Geometry check sheet. Reference: the model listing, model coordinates, mm. A direction names the side the tool comes from. Round coordinates to 2 decimals unless told otherwise and drop trailing zeros. Write each loop counter-clockwise with the first axis right and the second up, starting at its lowest first coordinate (ties: lowest second). Pieces come first, ordered by that corner, then holes. Notation, with made-up numbers: M 48.5,79 L 73.5,79 A20 cw 73.5,94 Z; hole C -8,20 d5. An arc over 180 degrees is marked long. One line per item, written item: value. Start each with the question number.
1. Depth check by flat-ended pin: P1, Ø1.5, axis at y = 24, z = 2.5, coming from the +X side; P2, Ø1.5, axis at y = 36.5, z = 1, coming from the -X side; P3, Ø2, axis at x = 2.5, z = 2, coming from the +Y side. Enter the tip coordinate at first touch or a pass-through.
2. Section check A-A (z = 1.9). Count the separate pieces of the cut face and the enclosed holes in it, and give its area (3 significant figures).
3. Release check for a two-part mould opening along X. For faces 4 (the cylindrical face through (-14.492, 20.606, 1.972)), 5 (the flat face through (0, -7, 2)), 6 (the cylindrical face through (-7.364, 86.072, 1.972)) record: pulls with the +X half, pulls with the -X half, needs draft (parallel to the pull), parting line crosses it, or undercut.
4. Section check C-C (x = -15.5). Record the boundary of the cut face in (y, z).
5. Access from +Z, -Z, +X, -X, +Y, -Y to the whole of each face (thin tool, end or side, straight path). Record for faces 1 (the cylindrical face through (9.16, 8.95, 1.97)), 2 (the cylindrical face through (-13.47, 81.37, 1.97)), 3 (the flat face through (0, 40, 0)).
6. Scan lines: probe 1 along Y at (x, z) = (-13, 1.8); probe 2 along Y at (x, z) = (4, 1.2); probe 3 along X at (y, z) = (26, 2.2). Record each from-to range of solid material in increasing order. Write a range as [from, to].
7. Section check D-D (y = 62). Record the boundary of the cut face in (x, z), and give its area (3 significant figures).
8. Section check B-B (y = 9.5). Record the boundary of the cut face in (x, z), and give its area (3 significant figures).
from build123d import *

# Parameters (mm, degrees)
SKETCH_1_R          = 3
SKETCH_1_R_2        = 7.5
SKETCH_1_R_3        = 6
EXTRUDE_1_DEPTH     = 4
CUT_EXTRUDE_START   = -10
CUT_EXTRUDE_2_DEPTH = 10
CUT_EXTRUDE_6_DEPTH = 10
FILLET_8_R          = 3
FILLET_9_R          = 10


with BuildPart() as part:
    # 草图1 → 凸台-拉伸1 (new body)
    with BuildSketch(Plane.XY):
        with BuildLine():
            Line((-39.588006912, 70.159203728), (-18.211604838, -1.988557391))
            ThreePointArc((-18.211604838, -1.988557391), (-15.688084184, -5.608917085), (-11.5, -7))
            Line((-11.5, -7), (11.5, -7))
            ThreePointArc((11.5, -7), (16.566581898, -4.83008777), (18.492010075, 0.334357752))
            Line((18.492010075, 0.334357752), (14.982878733, 73.716480896))
            ThreePointArc((14.982878733, 73.716480896), (9.406006267, 84.684478854), (-2.5, 87.790199458))
            Line((-2.5, 87.790199458), (-31.666666667, 82.860132972))
            ThreePointArc((-31.666666667, 82.860132972), (-38.485005613, 78.291944798), (-39.588006912, 70.159203728))
        make_face()
        with Locations((11.5, 0)):
            Circle(SKETCH_1_R, mode=Mode.SUBTRACT)
        with Locations((-11.5, 0)):
            Circle(SKETCH_1_R, mode=Mode.SUBTRACT)
        with Locations((0, 73)):
            Circle(SKETCH_1_R_2, mode=Mode.SUBTRACT)
        with Locations((-30, 73)):
            Circle(SKETCH_1_R_3, mode=Mode.SUBTRACT)
    extrude(amount=EXTRUDE_1_DEPTH)

    # 草图3 → 切除-拉伸2 (cut)
    with BuildSketch(Plane.XY.offset(4).offset(CUT_EXTRUDE_START)):
        with BuildLine():
            Line((-22.294207695, 79.373442159), (-12.695653982, 80.995893861))
            ThreePointArc((-12.695653982, 80.995893861), (-8.463678603, 85.388708293), (-2.832841434, 87.733938987))
            Line((-2.832841434, 87.733938987), (-31.666666667, 82.860132972))
            ThreePointArc((-31.666666667, 82.860132972), (-26.513309187, 82.372458972), (-22.294207695, 79.373442159))
        make_face()
    extrude(amount=CUT_EXTRUDE_2_DEPTH, mode=Mode.SUBTRACT)

    # 草图7 → 切除-拉伸6 (cut)
    with BuildSketch(Plane.XY.offset(4)):
        Polygon((3.295515487, 61), (-28.530502179, 61), (-14.691197263, 14.290789455), align=None)
        Polygon((10.116297473, 8), (8.055325934, 51.098548475), (-8.540998481, 8), align=None)
    extrude(amount=-CUT_EXTRUDE_6_DEPTH, mode=Mode.SUBTRACT)

    # 圆角8
    fillet_8_edges = [part.edges().sort_by_distance(p)[0] for p in [
        (8.055325934, 51.098548475, 2),
        (10.116297473, 8, 2),
        (-8.540998481, 8, 2),
        (3.295515487, 61, 2),
        (-14.691197263, 14.290789455, 2),
        (-28.530502179, 61, 2),
    ]]
    fillet(fillet_8_edges, radius=FILLET_8_R)

    # 圆角9
    # the kernel refuses this fillet: 10 mm, written as the material it adds along each edge
    with BuildSketch(Plane(origin=(-12.695653982, 80.995893861, 0), x_dir=(0.613787273879612, 0.789471457636965, 0), z_dir=(0, 0, 1))) as fillet_9_piece_1:
        with BuildLine():
            CenterArc((3.946152578, 9.951236707), FILLET_9_R, 227.457922435, 36.881499563)
            Line((-2.815162182, 2.583426808), (0, 0))
            ThreePointArc((0, 0), (1.479900866, 0.073163458), (2.959801732, 0))
        make_face()
    extrude(amount=4)
    with BuildSketch(Plane(origin=(-22.294207695, 79.373442159, 0), x_dir=(0.9860132971832692, 0.16666666666666718, 0), z_dir=(0, 0, 1))) as fillet_9_piece_2:
        with BuildLine():
            CenterArc((4.568502517, 10), FILLET_9_R, 228.590377891, 41.409622109)
            ThreePointArc((-2.04587576, 2.5), (-0.921320126, 1.33315892), (0, 0))
            Line((0, 0), (4.568502517, 0))
        make_face()
    extrude(amount=4)
    # the kernel refuses this fillet: 10 mm, written as the material it takes off along each edge
    with BuildSketch(Plane(origin=(-2.832841434, 87.733938987, -0.617519745), x_dir=(0.9860132971832704, 0.16666666666666025, 0), z_dir=(0, 0, 1))) as fillet_9_2_piece_1:
        with BuildLine():
            CenterArc((0.14264617, -10), FILLET_9_R, 90, 2.232449915)
            ThreePointArc((-0.246891263, -0.007589851), (-0.123461251, -0.003286845), (0, 0))
            Line((0, 0), (0.14264617, 0))
        make_face()
    extrude(amount=5.23503949, mode=Mode.SUBTRACT)


solid = part.part
Result sheet:
1. P1: stops at x = 17.4
1. P2: stops at x = -29.84
1. P3: stops at y = 87.92
2. separate pieces: 1
2. enclosed holes: 6
2. area: 2,750 mm2
3. face 4: undercut
3. face 5: needs draft
3. face 6: pulls with the -X half
4. outline: M -5.74,0 L 20.84,0 L 20.84,4 L -5.74,4 Z; M 61,0 L 80.57,0 L 80.57,4 L 61,4 Z
5. face 1: +Z, -Z
5. face 2: +Z, -Z, +Y
5. face 3: -Z, +X, -X, +Y, -Y
6. probe 1: y = [-6.84, -2.6], [2.6, 20.91], [61, 81.64]
6. probe 2: y = [-7, 8], [39.18, 66.66], [79.34, 87.46]
6. probe 3: x = [-26.5, -18.16], [-10.18, -1.61], [9.26, 17.26]
7. outline: M -37.17,0 L 15.54,0 L 15.54,4 L -37.17,4 Z
7. area: 211 mm2
8. outline: M -21.62,0 L -6.77,0 L -6.77,4 L -21.62,4 Z; M 9.57,0 L 18.05,0 L 18.05,4 L 9.57,4 Z
8. area: 93.3 mm2
